Autodesk Fusion 360 part; units mm, degrees
sketch "Sketch1" plane through (0, 0, 0) normal (1, 0, 0) x (0, 1, 0)
  line L0 (0, 0) -> (0, -40)
  line L1 (0, -40) -> (18.2, -40)
  line L2 (18.2, -40) -> (18.2, 30)
  line L3 (18.2, 30) -> (27.2, 30)
  line L4 (27.2, 30) -> (27.2, 48.65)
  line L5 (33.2, 48.6647) -> (77.2, 48.6647)
  line L6 (77.2, 48.6647) -> (77.2, 68.6647)
  line L7 (27.2, 48.65) -> (7.2, 48.65)
  line L8 (0, 0) -> (-8, 0)
  line L9 (-8, 0) -> (-8, -48)
  line L10 (-8, -48) -> (24.2, -48)
  line L11 (24.2, -48) -> (24.2, 2.6994)
  line L12 (33.2, 22) -> (33.2, 40.6647)
  line L13 (33.2, 40.6647) -> (33.2, 48.6647)
  line L14 (7.2, 48.65) -> (7.2, 54.65)
  line L15 (7.2, 54.65) -> (71.2, 54.65)
  line L16 (71.2, 54.65) -> (71.2, 68.6647)
  line L17 (71.2, 68.6647) -> (77.2, 68.6647)
  line L18 (33.2, 22) -> (24.2, 2.6994)
  line L19 (77.2, 48.6647) -> (24.2, -48)
  line L20 (70.3573, 48.6647) -> (24.2, -35.5199)
  line L21 (33.2, 40.6647) -> (39.2, 48.6647)
  dimension "d1" = 40
  dimension "d2" = 18.2
  dimension "d3" = 70
  dimension "d4" = 9
  dimension "d5" = 18.65
  dimension "d6" = 50
  dimension "d7" = 20
  dimension "d8" = 20
  dimension "d9" = 8
  dimension "d10" = 8
  dimension "d11" = 6
  dimension "d13" = 6
  dimension "d14" = 25
  dimension "d15" = 8
  dimension "d16" = 6
  dimension "d17" = 6
  dimension "d18" = 44
  dimension "d21" = 6
  dimension "d22" = 6
  dimension "d23" = 8
extrude "Extrude1" add sketch "Sketch1" along normal blind 22 contours L0 L1 L2 L3 L4 L5 L6 L7 L8 L9 L10 L11 L12 L13 L14 L15 L16 L17 L18 | L5 L11 L19 L20 | L5 L13 L21
Can you work these out from the model? Positions are in its coordinate system, mm. A direction names the side the tool comes from. Give positions to 0.01 mm unless a question says otherwise; leave off trailing zeros. Order: outer loops, then holes, each group sorted by start corner. A loop starts at its lowest first (then second) coordinate and runs counter-clockwise, first axis right, second up. Notation, with made-up numbers: M -32,67 L -3,67 A19 ccw -3,104 Z; hole C 4.5,41.5 d5. An arc over 180 degrees is marked long. Use a Markdown table: item, result. Add a question column.
Item 1: For faces 5 (the flat face through (11, 74, 68.665)), 6 (the flat face through (11, 23, 30)), 7 (the flat face through (10.85, 51.07, 1.01)), 8 (the flat face through (10.85, 36.16, 44.61)), 9 (the flat face through (11, 71.2, 62)), which set-ups out of +Z, -Z, +X, -X, +Y, -Y let a thin tool reach every point of the face, with its end or its side?
Item 2: If I drill on L1, parallel to Y at x = 19, z = -33.5; L2, parallel to Y at x = 13.75, z = -17; L3, parallel to Z at x = 18.5, y = 11.5, over which ranges is the centre line in solid material (lowest first)? Write a range as [from, to].
Item 3: We'd pull the mould along Y, two halves only. Please class faces 1 (the flat face through (10.85, 47.6, 7.16)), 2 (the flat face through (11, 0, -20)), 3 (the flat face through (11, 17, 48.65)), 4 (the flat face through (11, 7.2, 52)): +Y half, -Y half, draft (parallel to the pull), parting line (faces both ways), or undercut.
Item 4: Suppose I cut it at B-B (x = 9.25). List the corners of the cut face in (y, z) for me, then the cut area to 3 significant figures.
Item 5: Suppose I cut it at D-D (z = -21). List the corners of the cut face in (x, y) for me, then the cut area to 3 significant figures.
Item 6: Will these pins go through, and if not, where does the flat tip stop? pin 1 (4 mm diameter, centred on x = 10, y = 49, fed in from +Z); pin 2 (5.5 mm diameter, centred on x = 6.5, z = 42.5, fed in from -Y); pin 3 (6.5 mm diameter, centred on x = 15, z = -24, fed in from +Y).
Item 7: Suppose I cut it at C-C (z = 38.5). List the corners of the cut face in (x, y) for me.
Item 8: Suppose I cut it at A-A (y = 20). List the corners of the cut face in (x, z) for me.
Answer sheet:
| question | item | result |
|---|---|---|
| 1 | face 5 | +Z, +X, -X, +Y, -Y |
| 1 | face 6 | +X, -X, -Y |
| 1 | face 7 | -Z, +X, -X, +Y |
| 1 | face 8 | +X, -X |
| 1 | face 9 | +Z, +X, -X, -Y |
| 2 | L1 | y = [-8, 0], [18.2, 24.2], [25.31, 32.15] |
| 2 | L2 | y = [-8, 0], [18.2, 24.2], [34.35, 41.2] |
| 2 | L3 | z = [-48, -40], [48.65, 54.65] |
| 3 | face 1 | undercut |
| 3 | face 2 | undercut |
| 3 | face 3 | draft |
| 3 | face 4 | -Y half |
| 4 | outline | M -8,-48 L 24.2,-48 L 77.2,48.66 L 77.2,68.66 L 71.2,68.66 L 71.2,54.65 L 7.2,54.65 L 7.2,48.65 L 27.2,48.65 L 27.2,30 L 18.2,30 L 18.2,-40 L 0,-40 L 0,0 L -8,0 Z; hole M 24.2,-35.52 L 70.36,48.66 L 39.2,48.66 L 33.2,40.66 L 33.2,22 L 24.2,2.7 Z |
| 4 | area | 2,410 mm² |
| 5 | outline | M 0,-8 L 22,-8 L 22,0 L 0,0 Z; M 0,18.2 L 22,18.2 L 22,24.2 L 0,24.2 Z; M 0,32.16 L 22,32.16 L 22,39 L 0,39 Z |
| 5 | area | 459 mm² |
| 6 | pin 1 | stops at z = 54.65 |
| 6 | pin 2 | stops at y = 27.2 |
| 6 | pin 3 | stops at y = 39.14 |
| 7 | outline | M 0,27.2 L 22,27.2 L 22,33.2 L 0,33.2 Z; M 0,64.78 L 22,64.78 L 22,71.63 L 0,71.63 Z |
| 8 | outline | M 0,-48 L 22,-48 L 22,30 L 0,30 Z; M 0,48.65 L 22,48.65 L 22,54.65 L 0,54.65 Z |
